Part model, mm, in its own coordinate system. A direction names the side the tool comes from. Round coordinates to 2 decimals unless told otherwise and drop trailing zeros. Write each loop counter-clockwise with the first axis right and the second up, starting at its lowest first coordinate (ties: lowest second). Pieces come first, ordered by that corner, then holes. Notation, with made-up numbers: M 73,73 L 109,73 A33 cw 109,110 Z; hole C 9,76 d11. An arc over 180 degrees is marked long. Answer as a JSON object with one key per item and string values. Group by question number.
1. Drill centre lines: line 1 (Z direction, x = -22.5, y = 21.5); line 2 (X direction, y = -19, z = 6); line 3 (X direction, y = -28, z = 14). Where is each one in solid material? Low to high. Write a range as from..to.
2. Band-saw the part on B-B, the plane y = 0. Write the cut outline in (x, z) (3 decimals).
3. Drop flat-ended pins along their axis: pin 1 (4 mm diameter, centred on x = -41.28, y = 23.83, fed in from +Z); pin 2 (3.5 mm diameter, centred on x = -0.5, y = -47, fed in from -Z); pin 3 (6 mm diameter, centred on x = 37.5, z = 13.5, fed in from +Y). Give the stop position or say it passes through.
4. Which spindle directions (+Z, -Z, +X, -X, +Y, -Y) get a long thin tool onto all of the face, cutting with end or side? Do faces 4 (the face through (2, -48, 17.5)), 5 (the face through (-40.24, 25.83, 10.07)). Say none if no direction does.
5. Two-plate mould, pull along Y, no slides. Class faces 1 (the face through (14.32, -64.46, 13.9)), 2 (the face through (1, 1, 15)), 3 (the face through (-1, 1, 18)): +Y half, -Y half, draft (parallel to the pull), parting line (faces both ways), or undercut.
6. Band-saw the part on A-A, the plane z = 11. Write the cut outline in (x, y), plus the area to 3 significant figures.
from build123d import *

# Parameters (mm, degrees)
F2_R     = 2.25
F2_R_2   = 1.65
F3_DEPTH = 10
F4_R     = 1.65
F5_DEPTH = 3
F6_R     = 2.5
F7_DEPTH = 0.5


# Not quite as in the source:
# - ends of sketch curves that miss each other by under 0.0002 mm in the source are joined


with BuildPart() as f1:
    # F0 (on Front) → F1 (revolve)
    with BuildSketch(Plane.XZ):
        with BuildLine():
            Line((0, 15.0000001043), (0, 18))
            Line((0, 18), (-60, 18))
            ThreePointArc((-60, 18), (-63.175, 17.149261314), (-65.499261314, 14.825))
            Line((-65.499261314, 14.825), (-74.0584790548, 0))
            ThreePointArc((-74.0584790548, 0), (-73.5094409491, -2.0490381057), (-71.4604028434, -1.5))
            Line((-71.4604028434, -1.5), (-62.901185193, 13.3250000522))
            ThreePointArc((-62.901185193, 13.3250000522), (-61.6750000522, 14.551185193), (-60, 15.0000001043))
            Line((-60, 15.0000001043), (0, 15.0000001043))
        make_face()
    revolve(axis=Axis((0, 0, 16.5000000522), (0, 0, -1)))

    # F2 (on face) → F3 (join)
    with BuildSketch(Plane(origin=(0, 0, 15.0000001043), x_dir=(1, 0, 0), z_dir=(0, 0, -1))):
        with Locations((0, 47.6650122409)):
            Circle(F2_R)
        with Locations((0, 47.6650122409)):
            Circle(F2_R_2, mode=Mode.SUBTRACT)
        with Locations((-41.2791114723, -23.8325061204)):
            Circle(F2_R)
        with Locations((-41.2791114723, -23.8325061204)):
            Circle(F2_R_2, mode=Mode.SUBTRACT)
        with Locations((41.2791114723, -23.8325061204)):
            Circle(F2_R)
        with Locations((41.2791114723, -23.8325061204)):
            Circle(F2_R_2, mode=Mode.SUBTRACT)
    extrude(amount=F3_DEPTH)

    # F4 (on face) → F5 (cut)
    with BuildSketch(Plane(origin=(0, 0, 15.0000001043), x_dir=(1, 0, 0), z_dir=(0, 0, -1))):
        with Locations((0, 47.6650122409)):
            Circle(F4_R)
        with Locations((-41.2791114723, -23.8325061204)):
            Circle(F4_R)
        with Locations((41.2791114723, -23.8325061204)):
            Circle(F4_R)
    extrude(amount=-F5_DEPTH, mode=Mode.SUBTRACT)

    # F6 (on face) → F7 (cut)
    with BuildSketch(Plane.XY.offset(18)):
        with Locations((0, -47.6650122409)):
            Circle(F6_R)
        with Locations((41.2791114723, 23.8325061204)):
            Circle(F6_R)
        with Locations((-41.2791114723, 23.8325061204)):
            Circle(F6_R)
    extrude(amount=-F7_DEPTH, mode=Mode.SUBTRACT)


solid = f1.part
Worked answers:
{
 "1": {"line 1": "z = 15..18", "line 2": "x = -67.99..-64.39, 64.39..67.99", "line 3": "x = -59.74..-55.75, 55.75..59.74"},
 "2": {"outline": "M -74.058,0 A1.5 ccw -71.46,-1.5 L -62.901,13.325 A3.35 cw -60,15 L 60,15 A3.35 cw 62.901,13.325 L 71.46,-1.5 A1.5 ccw 74.058,0 L 65.499,14.825 A6.35 ccw 60,18 L -60,18 A6.35 ccw -65.499,14.825 Z"},
 "3": {"pin 1": "stops at z = 17.5", "pin 2": "stops at z = 5", "pin 3": "stops at y = 57.48"},
 "4": {"face 4": "+Z", "face 5": "-Z"},
 "5": {"face 1": "parting line", "face 2": "undercut", "face 3": "draft"},
 "6": {"outline": "C 0,0 d135.42; C -41.28,23.83 d4.5; C 0,-47.67 d4.5; C 41.28,23.83 d4.5; hole C 0,0 d128.49; hole C -41.28,23.83 d3.3; hole C 0,-47.67 d3.3; hole C 41.28,23.83 d3.3", "area": "1,460 mm^2"}
}
